Print and shaded views of the part. All mm, measured from the part's lowest x, y and z. A direction names the side the tool comes from. Round coordinates to 2 decimals unless told otherwise and drop trailing zeros. Loops run counter-clockwise (first coordinate to the right, second up) from the corner with the lowest first, then second, coordinate; pieces in that order, holes last. Notation, with made-up numbers: (-35.5, -28.5) - (-17.5, -28.5) arc R22 ccw to (-17.5, -10.5) - close; hole circle Ø9 at (17, -6). An arc over 180 degrees is marked (long way). Answer as a JSON object with one key per item and string values.
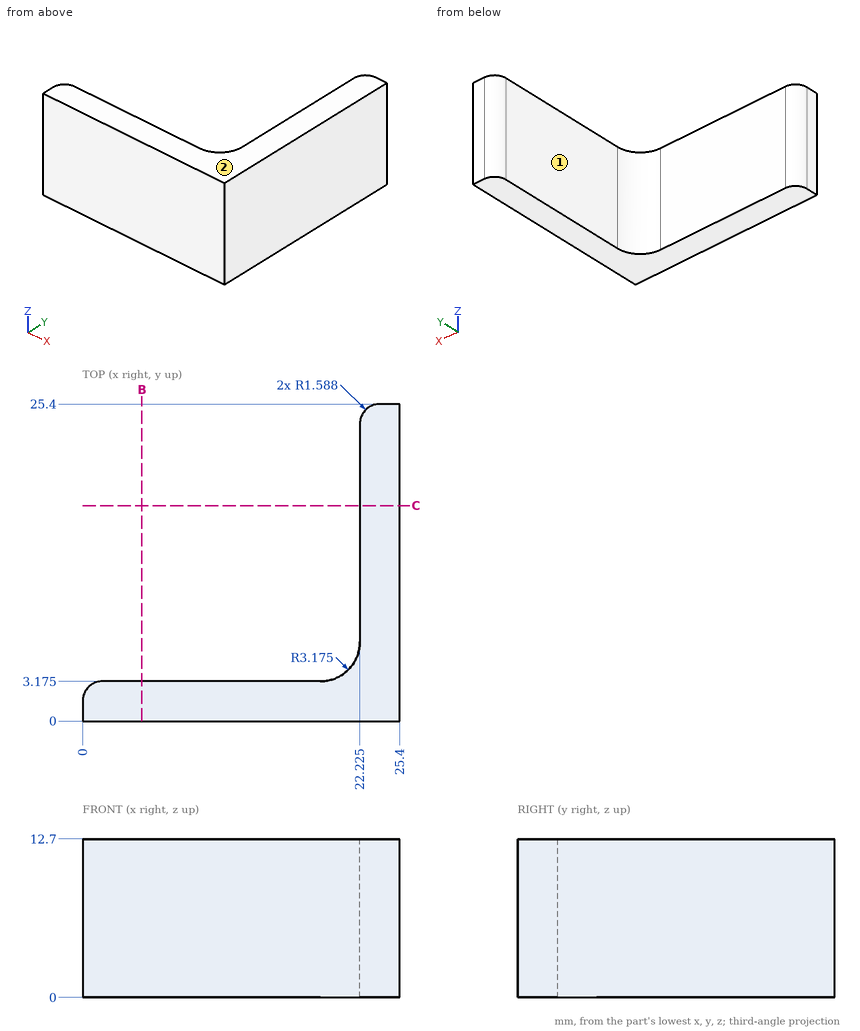
1) Probe probe 1 along X at (y, z) = (9.75, 12.25) (1 decimal); probe 2 along Y at (x, z) = (12.25, 8) (1 decimal); probe 3 along X at (y, z) = (2, 8.25) (1 decimal). List the from-to ranges inside material, lowest first.
Values follow:
{"probe 1": "22.2 to 25.4", "probe 2": "0 to 3.2", "probe 3": "0.1 to 25.4"}
2) Slice it at C-C on y = 17.25. List the corners of the cut face in (x, z) (1 decimal).
Values follow:
{"outline": "(22.2, 0) - (25.4, 0) - (25.4, 12.7) - (22.2, 12.7) - close"}
3) Tool access for the marked faces 1 and 2: list every direction of +Z, -Z, +X, -X, +Y, -Y with a clear straight run to the whole face (end or side of a thin tool).
Values follow:
{"face 1": "+Z, -Z, -X, +Y", "face 2": "+Z, +X, -X, +Y, -Y"}
4) Slice it at B-B on x = 4.75. List the corners of the cut face in (y, z) (1 decimal).
Values follow:
{"outline": "(0, 0) - (3.2, 0) - (3.2, 12.7) - (0, 12.7) - close"}
5) Drop flat-ended pins along their axis: P1, Ø5, axis at x = 5.5, z = 9, coming from the +Y side (1 decimal); P2, Ø4, axis at y = 11.5, z = 7.5, coming from the -X side (1 decimal). Give the stop position or say it passes through.
Values follow:
{"P1": "y = 3.2", "P2": "x = 22.2"}
